The model under review builds one solid part; all positions refer to its coordinate system, in mm. Round coordinates to 2 decimals unless told otherwise and drop trailing zeros. Write each loop counter-clockwise with the first axis right and the second up, starting at its lowest first coordinate (ties: lowest second). Pieces come first, ordered by that corner, then holes. Notation, with made-up numbers: M 74,76.5 L 117,76.5 A16 ccw 117,102.5 Z; hole C 76,-39.75 d8. An arc over 180 degrees is marked long. Write item = value, one per line. Start each with the question number.
Item 1: Take a section at A-A, the plane x = 8. Give the boundary of the cut face in (y, z).
Item 2: Take a section at B-B, the plane y = 118. Give the boundary of the cut face in (x, z).
Item 3: To check wall thickness, follow line 1 along Y through (x, z) = (8, 9.5); line 2 along Z through (x, y) = (1.75, 110); line 3 along X through (y, z) = (123, 6.5). State the ranges of each line that lie inside material, in increasing order.
Item 4: For pin 1 Ø1 at (x, y) = (10.5, 152) entering from -Z; pin 2 Ø3.5 at (x, y) = (8, 94) entering from +Z; pin 3 Ø0.6 at (x, y) = (2.5, 196) entering from -Z, all flat-tipped, find the tip position at first contact; note any pin that passes through.
Item 5: Take a section at C-C, the plane z = 2. Give the boundary of the cut face in (x, y).
Item 6: The part is to be moulded in two halves that separate along X. For faces 1 (the cylindrical face through (7.52, 38.67, 9.26)), 2 (the flat face through (16, 136, 5)), 3 (the flat face through (7, 275, 9)), 4 (the flat face through (8, 139, 8.5)), say which applies: +X half, -X half, draft (parallel to the pull), parting line (faces both ways), or undercut.
Item 7: Take a section at D-D, the plane y = 166. Give the boundary of the cut face in (x, z).
from build123d import *

# Parameters (mm, degrees)
SKETCH1_W           = 16
SKETCH1_H           = 10
BOSS_EXTRUDE1_DEPTH = 275
CUT_EXTRUDE1_DEPTH  = 275
SKETCH3_R           = 2.9
SKETCH3_R_2         = 3.7
CUT_EXTRUDE2_DEPTH  = 276.646512766


with BuildPart() as part:
    # Sketch1 → Boss-Extrude1 (new body)
    with BuildSketch(Plane(origin=(0, 0, 0), x_dir=(1, 0, 0), z_dir=(0, 1, 0))):
        with Locations((8, -5)):
            Rectangle(SKETCH1_W, SKETCH1_H)
    extrude(amount=BOSS_EXTRUDE1_DEPTH)

    # Sketch2 → Cut-Extrude1 (cut)
    with BuildSketch(Plane(origin=(0, 275, 0), x_dir=(1, 0, 0), z_dir=(0, 1, 0))):
        Polygon((1.5, 0), (1.5, -3.5), (3.5, -3.5), (3.5, -5), (1.5, -5), (1.5, -8.5), (14.5, -8.5), (14.5, -5), (12.5, -5), (12.5, -3.5), (14.5, -3.5), (14.5, 0), align=None)
    extrude(amount=-CUT_EXTRUDE1_DEPTH, mode=Mode.SUBTRACT)

    # Sketch3 → Cut-Extrude2 (cut, through all)
    with BuildSketch(Plane.XY.offset(10)):
        with Locations((8, 15.5)):
            Circle(SKETCH3_R)
        with Locations((8, 35)):
            Circle(SKETCH3_R_2)
        with Locations((8, 94)):
            Circle(SKETCH3_R)
        with Locations((8, 118)):
            Circle(SKETCH3_R_2)
    extrude(amount=-CUT_EXTRUDE2_DEPTH, mode=Mode.SUBTRACT)


solid = part.part
Response values:
q1.outline = M 0,8.5 L 12.6,8.5 L 12.6,10 L 0,10 Z; M 18.4,8.5 L 31.3,8.5 L 31.3,10 L 18.4,10 Z; M 38.7,8.5 L 91.1,8.5 L 91.1,10 L 38.7,10 Z; M 96.9,8.5 L 114.3,8.5 L 114.3,10 L 96.9,10 Z; M 121.7,8.5 L 275,8.5 L 275,10 L 121.7,10 Z
q2.outline = M 0,0 L 1.5,0 L 1.5,3.5 L 3.5,3.5 L 3.5,5 L 1.5,5 L 1.5,8.5 L 4.3,8.5 L 4.3,10 L 0,10 Z; M 11.7,8.5 L 14.5,8.5 L 14.5,5 L 12.5,5 L 12.5,3.5 L 14.5,3.5 L 14.5,0 L 16,0 L 16,10 L 11.7,10 Z
q3.line_1 = 0 to 12.6, 18.4 to 31.3, 38.7 to 91.1, 96.9 to 114.3, 121.7 to 275
q3.line_2 = 3.5 to 5, 8.5 to 10
q3.line_3 = 0 to 1.5, 14.5 to 16
q4.pin_1 = 8.5
q4.pin_2 = through
q4.pin_3 = 3.5
q5.outline = M 0,0 L 1.5,0 L 1.5,275 L 0,275 Z; M 14.5,0 L 16,0 L 16,275 L 14.5,275 Z
q6.face_1 = undercut
q6.face_2 = +X half
q6.face_3 = draft
q6.face_4 = undercut
q7.outline = M 0,0 L 1.5,0 L 1.5,3.5 L 3.5,3.5 L 3.5,5 L 1.5,5 L 1.5,8.5 L 14.5,8.5 L 14.5,5 L 12.5,5 L 12.5,3.5 L 14.5,3.5 L 14.5,0 L 16,0 L 16,10 L 0,10 Z
